from build123d import *

# Parameters (mm, degrees)
CYLINDER1981_R     = 2.6
CYLINDER1981_DEPTH = 33
CYLINDER1980_R     = 13.25
CYLINDER1980_DEPTH = 2
CHAMFER100_SIZE    = 1


with BuildPart() as obj1:
    # Cylinder1981 → Cylinder1981 (new body)
    with BuildSketch(Plane.XY.offset(42)):
        Circle(CYLINDER1981_R)
    extrude(amount=CYLINDER1981_DEPTH)


with BuildPart() as chamfer100:
    # Cylinder1980 → Cylinder1980 (new body)
    with BuildSketch(Plane.XY.offset(46.65)):
        Circle(CYLINDER1980_R)
    extrude(amount=CYLINDER1980_DEPTH)

    # Cut740: cut obj1
    add(obj1.part, mode=Mode.SUBTRACT)

    # Chamfer100
    chamfer100_edges = [chamfer100.edges().sort_by_distance(p)[0] for p in [
        (-13.25, 0, 46.65),
    ]]
    chamfer(chamfer100_edges, length=CHAMFER100_SIZE)


solid = chamfer100.part
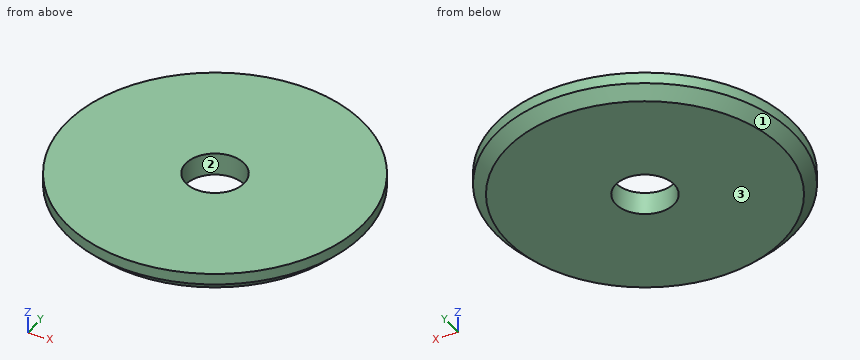
Here's how the part is built. I have some questions about the finished solid (model axes, mm). Face numbers are marked on the shaded views. Coordinates: 2 decimals unless noted, no trailing zeros. Order: outer loops, then holes, each group sorted by start corner. A loop starts at its lowest first (then second) coordinate and runs counter-clockwise, first axis right, second up. Notation, with made-up numbers: (41.25, 57.5) -> (95.25, 57.5) arc R16 ccw to (95.25, 82.5) -> close; hole circle Ø5 at (88, 2.25). An arc over 180 degrees is marked (long way). Answer in a Markdown table with one row per item.
(1) I want a section at A-A on x = 0. List the corners of the cut face in (y, z) for me, then the cut area to 3 significant figures.
Answer key:
| item | result |
|---|---|
| outline | (-13.25, 47.65) -> (-12.25, 46.65) -> (-2.6, 46.65) -> (-2.6, 48.65) -> (-13.25, 48.65) -> close; (2.6, 46.65) -> (12.25, 46.65) -> (13.25, 47.65) -> (13.25, 48.65) -> (2.6, 48.65) -> close |
| area | 41.6 mm^2 |
(2) Please list where these lines run through material, in increasing order: probe 1 along Y at (x, z) = (0, 48.1); probe 2 along Y at (x, z) = (0, 47.35); probe 3 along X at (y, z) = (0.75, 47.3).
Answer key:
| item | result |
|---|---|
| probe 1 | -13.25 to -2.6, 2.6 to 13.25 |
| probe 2 | -12.95 to -2.6, 2.6 to 12.95 |
| probe 3 | -12.88 to -2.49, 2.49 to 12.88 |
(3) Thinking about a two-plate mould opening in Y: for the marked faces 1, 2 and 3, which applies, +Y half, -Y half, draft (parallel to the pull), parting line (faces both ways), or undercut?
Answer key:
| item | result |
|---|---|
| face 1 | parting line |
| face 2 | undercut |
| face 3 | draft |
(4) I want a section at C-C on z = 47.05. List the corners of the cut face in (x, y) for me, then the cut area to 3 significant figures.
Answer key:
| item | result |
|---|---|
| outline | circle Ø25.3 at (0, 0); hole circle Ø5.2 at (0, 0) |
| area | 481 mm^2 |
